from build123d import *

# Parameters (mm, degrees)
SKETCH1_W           = 132
SKETCH1_H           = 82
BOSS_EXTRUDE1_DEPTH = 11
SKETCH2_W           = 112
SKETCH2_H           = 82
BOSS_EXTRUDE2_DEPTH = 43
SKETCH3_R           = 6
CUT_EXTRUDE1_DEPTH  = 112
SCALE1_SCALE        = 0.1


with BuildPart() as part:
    # Sketch1 → Boss-Extrude1 (new body)
    with BuildSketch(Plane(origin=(0, 0, 0), x_dir=(1, 0, 0), z_dir=(0, 1, 0))):
        with Locations((-48.872246696, 7.585903084)):
            Rectangle(SKETCH1_W, SKETCH1_H)
    extrude(amount=BOSS_EXTRUDE1_DEPTH)

    # Sketch2 → Boss-Extrude2 (add)
    with BuildSketch(Plane(origin=(0, 11, 0), x_dir=(1, 0, 0), z_dir=(0, 1, 0))):
        with Locations((-48.872246696, 7.585903084)):
            Rectangle(SKETCH2_W, SKETCH2_H)
    extrude(amount=BOSS_EXTRUDE2_DEPTH)

    # Sketch3 → Cut-Extrude1 (cut)
    with BuildSketch(Plane(origin=(7.127753304, 0, 0), x_dir=(0, 0, -1), z_dir=(1, 0, 0))):
        with Locations((-13.414096916, 43)):
            Circle(SKETCH3_R)
        with Locations((27.585903084, 43)):
            Circle(SKETCH3_R)
    extrude(amount=-CUT_EXTRUDE1_DEPTH, mode=Mode.SUBTRACT)


with BuildPart() as part_1:
    # Scale1: scaled about (-48.872246696, 25.376724614, -7.611825736)
    add(part.part.scale(SCALE1_SCALE).moved(Location((-43.985022026, 22.839052153, -6.850643162))))


solid = part_1.part
Geometry: final body of the model. Coordinates: model frame, mm. A direction names the side the tool comes from. Give positions to 0.01 mm unless a question says otherwise; leave off trailing zeros. Write each loop counter-clockwise with the first axis right and the second up, starting at its lowest first coordinate (ties: lowest second). Pieces come first, ordered by that corner, then holes. Notation, with made-up numbers: (-7, 73) - (5, 73) arc R17 cw to (5, 78) - close; hole circle Ø5 at (67.5, 61.25). An arc over 180 degrees is marked (long way). Return JSON: item names as keys, results as strings. Group by question number.
1) Mould query, pull axis Z, two halves, no side actions, for faces 1 (the cylindrical face through (-48.79, 27.32, -6.08)), 2 (the flat face through (-49, 26, -3.509)), 3 (the flat face through (-55, 23.939, -8)). Classes: released by +Z, released by -Z, zero draft, split by the parting line, or undercut.
2) Section C-C on x = -53.25. Return the cut outline in (y, z), plus the area to 3 significant figures.
3) Section A-A on z = -10.75. Return the cut outline in (x, y), plus the area to 3 significant figures.
4) First-contact query: P1, Ø2, axis at y = 25.5, z = -6.5, coming from the -X side; P2, Ø1, axis at y = 27, z = -5, coming from the +X side; P3, Ø0.5, axis at x = -54.5, z = -6, coming from the +Y side; P4, Ø0.5, axis at x = -42.5, z = -6, coming from the +Y side. Flat tips, straight axial feed; report the tip coordinate or a pass-through.
5) Line query: line 1 (Z direction, x = -47.25, y = 26.85); line 2 (X direction, y = 26.2, z = -11); line 3 (Y direction, x = -46.5, z = -9.25). Output: solid intervals per line, ascending.
6) Section D-D on z = -9.75. Return the cut outline in (x, y).
7) Set-up query: faces 4 (the flat face through (-49, 28.239, -8)), 5 (the flat face through (-54.472, 26, -8)), 6 (the flat face through (-43, 23.939, -8)). Return all of +Z, -Z, +X, -X, +Y, -Y with unobstructed straight access to the full face (end or side cutting, diameter ignored); none if empty.
8) Section B-B on y = 26.95. Return the cut outline in (x, z).
Filled in:
{
 "1": {"face 1": "undercut", "face 2": "released by +Z", "face 3": "zero draft"},
 "2": {"outline": "(22.84, -11.71) - (28.24, -11.71) - (28.24, -3.51) - (22.84, -3.51) - close; hole circle Ø1.2 at (27.14, -9.61); hole circle Ø1.2 at (27.14, -5.51)", "area": "42.0 mm^2"},
 "3": {"outline": "(-55.47, 22.84) - (-42.27, 22.84) - (-42.27, 23.94) - (-43.27, 23.94) - (-43.27, 28.24) - (-54.47, 28.24) - (-54.47, 23.94) - (-55.47, 23.94) - close", "area": "62.7 mm^2"},
 "4": {"P1": "stops at x = -54.47", "P2": "stops at x = -43.27", "P3": "stops at y = 28.24", "P4": "stops at y = 23.94"},
 "5": {"line 1": "z = -11.71 to -10.14, -9.08 to -6.04, -4.98 to -3.51", "line 2": "x = -54.47 to -43.27", "line 3": "y = 22.84 to 26.66, 27.62 to 28.24"},
 "6": {"outline": "(-55.47, 22.84) - (-42.27, 22.84) - (-42.27, 23.94) - (-43.27, 23.94) - (-43.27, 26.56) - (-54.47, 26.56) - (-54.47, 23.94) - (-55.47, 23.94) - close; (-54.47, 27.72) - (-43.27, 27.72) - (-43.27, 28.24) - (-54.47, 28.24) - close"},
 "7": {"face 4": "+Z, -Z, +X, -X, +Y", "face 5": "+Z, -Z, -X, +Y", "face 6": "+Z, -Z, +X, +Y"},
 "8": {"outline": "(-54.47, -11.71) - (-43.27, -11.71) - (-43.27, -10.18) - (-54.47, -10.18) - close; (-54.47, -9.04) - (-43.27, -9.04) - (-43.27, -6.08) - (-54.47, -6.08) - close; (-54.47, -4.94) - (-43.27, -4.94) - (-43.27, -3.51) - (-54.47, -3.51) - close"}
}
